Autodesk Inventor part; units mm, degrees
ref_plane "YZ Plane" through (0, 0, 0) normal (1, 0, 0) x (0, 1, 0)
ref_plane "XZ Plane" through (0, 0, 0) normal (0, 1, 0) x (-1, 0, 0)
ref_plane "XY Plane" through (0, 0, 0) normal (0, 0, 1) x (1, 0, 0)
sketch "Boceto1" plane through (0, 0, 0) normal (0, 0, 1) x (1, 0, 0)
  line L0 (-13.5, 62) -> (13.5, 62)
  line L1 (13.5, 62) -> (13.5, 0)
  line L2 (13.5, 0) -> (-13.5, 0)
  line L3 (-13.5, 0) -> (-13.5, 62)
  line L4 (0, 0) -> (0, 62) construction
  line L5 (0, 40.815) -> (8.5, 35.9075)
  line L6 (8.5, 35.9075) -> (8.5, 26.0925)
  line L7 (8.5, 26.0925) -> (0, 21.185)
  line L8 (0, 21.185) -> (-8.5, 26.0925)
  line L9 (-8.5, 26.0925) -> (-8.5, 35.9075)
  line L10 (-8.5, 35.9075) -> (0, 40.815)
  line L11 (-8.5, 35.9075) -> (-13.5, 35.9075) construction
  line L12 (8.5, 35.9075) -> (13.5, 35.9075) construction
  point P0 (0, 31)
  dimension "d20" = 17
  dimension "d21" = 5
  dimension "d22" = 27
  dimension "d23" = 62
extrude "Extrusión1" add sketch "Boceto1" along normal blind 6
sketch "Boceto2" plane through (0, 0, 0) normal (0, 0, -1) x (-1, 0, 0)
  line L0 (-8.5, 26.0925) -> (-8.5, 35.9075)
  line L1 (-8.5, 35.9075) -> (0, 40.815)
  line L2 (0, 40.815) -> (8.5, 35.9075)
  line L3 (8.5, 35.9075) -> (8.5, 26.0925)
  line L4 (8.5, 26.0925) -> (0, 21.185)
  line L5 (0, 21.185) -> (-8.5, 26.0925)
  line L6 (13.5, 62) -> (-13.5, 62)
  line L7 (-13.5, 62) -> (-13.5, 0)
  line L8 (-13.5, 0) -> (13.5, 0)
  line L9 (13.5, 0) -> (13.5, 62)
  point P0 (0, 0)
extrude "Extrusión2" add sketch "Boceto2" along normal blind 6 contours L0 L1 L2 L3 L4 L5 | L9 L8 L7 L6
sketch "Boceto3" plane through (0, 0, -6) normal (0, 0, -1) x (-1, 0, 0)
  line L0 (0, 0) -> (0, 62) construction
  line L1 (-13.5, 62) -> (13.5, 62)
  circle A0 centre (0, 31) radius 5.5
  dimension "d18" = 11
extrude "Extrusión3" cut sketch "Boceto3" against normal up to next
sketch "Boceto5" plane through (0, 0, 6) normal (0, 0, 1) x (1, 0, 0)
  line L0 (-13.5, 0) -> (-13.5, 62)
  line L1 (13.5, 62) -> (13.5, 0)
  line L2 (-13.5, 0) -> (13.5, 0)
  line L3 (13.5, 0) -> (13.5, 12)
  line L4 (13.5, 12) -> (-13.5, 12)
  line L5 (-13.5, 12) -> (-13.5, 0)
  line L6 (13.5, 62) -> (-13.5, 62)
  line L7 (-13.5, 62) -> (13.5, 62)
  line L8 (13.5, 62) -> (13.5, 50)
  line L9 (13.5, 50) -> (-13.5, 50)
  line L10 (-13.5, 50) -> (-13.5, 62)
  line L11 (-17.3027, 31) -> (12.0796, 31) construction
  line L12 (-8.5, 26.0925) -> (-8.5, 35.9075)
  point P0 (0, 0)
  point P1 (-8.5, 31)
  dimension "d24" = 12
extrude "Extrusión4" add sketch "Boceto5" along normal blind 115 contours L0 L4 L1 L2 | L0 L6 L1 L9
sketch "Boceto9" plane through (-13.5, 0, -6) normal (0, -1, 0) x (1, 0, 0)
  circle A0 centre (13.5, 110) radius 5
  line L0 (0, 127) -> (27, 127)
  line L1 (13.5, 110) -> (13.5, 115)
  line L2 (13.5, 115) -> (13.5, 127)
  line L3 (0, 127) -> (27, 127)
  point P0 (13.5, 6)
  dimension "d25" = 10
  dimension "d32" = 12
extrude "Extrusión8" cut sketch "Boceto9" against normal up to surface (12 mm away)
sketch "Boceto10" plane through (0, 0, -6) normal (0, 0, -1) x (-1, 0, 0)
  circle A0 centre (0, 31) radius 11
  circle A1 centre (0, 31) radius 5.5
  point P0 (0, 0)
  dimension "d29" = 22
extrude "Extrusión9" cut sketch "Boceto10" against normal blind 2.5
sketch "Boceto11" plane through (-13.5, 12, 6) normal (0, 1, 0) x (1, 0, 0)
  line L0 (21.5, -106) -> (5.5, -106) construction
  line L1 (5.5, -106) -> (5.5, -90) construction
  line L2 (5.5, -90) -> (21.5, -90) construction
  line L3 (21.5, -90) -> (21.5, -106) construction
  line L4 (5.5, -106) -> (21.5, -90) construction
  circle A0 centre (13.5, -98) radius 8 construction
  circle A1 centre (13.5, -98) radius 11.3137
  line L5 (27, 0) -> (27, -115)
  circle A2 centre (13.5, -98) radius 5
  point P0 (13.5, 6)
  dimension "d45" = 16
extrude "Extrusión10" cut sketch "Boceto11" against normal blind 3 contours A1 | A2
sketch "Boceto12" plane through (-13.5, 0, -6) normal (0, -1, 0) x (1, 0, 0)
  circle A0 centre (13.5, 110) radius 11.3137
  line L0 (0, 127) -> (0, 0)
  point P0 (13.5, 6)
extrude "Extrusión11" cut sketch "Boceto12" against normal blind 3
sketch "Boceto14" plane through (-13.5, 62, -6) normal (0, 1, 0) x (1, 0, 0)
  circle A0 centre (13.5, -110) radius 5
  circle A1 centre (13.5, -110) radius 5
  point P0 (13.5, -6)
  dimension "d38" = 10
extrude "Extrusión12" cut sketch "Boceto14" against normal up to next
sketch "Boceto15" plane through (-13.5, 50, 6) normal (0, -1, 0) x (1, 0, 0)
  circle A0 centre (13.5, 98) radius 5
  circle A1 centre (13.5, 98) radius 12
  point P0 (13.5, -6)
  dimension "d41" = 24
extrude "Extrusión13" cut sketch "Boceto15" against normal blind 8
fillet "Empalme4" radius 12 4 edges at (13.5, 56, 121) (-13.5, 56, 121) (13.5, 6, 121) (-13.5, 6, 121)
fillet "Empalme5" radius 12 2 edges at (0, 0, -6) (0, 62, -6)
fillet "Empalme6" radius 12 2 edges at (0, 12, 6) (0, 50, 6)
CAD build for the part. Positions are in the model's coordinates, mm. A direction names the side the tool comes from. Round coordinates to 2 decimals unless told otherwise and drop trailing zeros. Write each loop counter-clockwise with the first axis right and the second up, starting at its lowest first coordinate (ties: lowest second). Pieces come first, ordered by that corner, then holes. Notation, with made-up numbers: M 31,47 L 57,47 A16 cw 57,74 Z; hole C -1.5,48 d9. An arc over 180 degrees is marked long. Use a Markdown table: item, result. Add a question column.
1. Drill centre lines: probe 1 along Y at (x, z) = (-5.5, 52.5); probe 2 along X at (y, z) = (10.05, 104); probe 3 along Y at (x, z) = (-1.5, 95). Where is each one in solid material? Low to high.
2. Slice it at C-C on z = 47.5. Give the cut face in (x, y).
3. Pull direction X, two halves, no side cores. Call faces 6 (the face through (-12, 31, -6)), 7 (the face through (-0.2, 58, 98.8)), 8 (the face through (-10.08, 56.08, 117.39)): released by +X, released by -X, zero draft, split by the parting line, or undercut.
4. Slice it at B-B on z = 104. Give the cut face in (x, y).
5. Flat gauge pins, fed straight in: P1, Ø7, axis at x = 5.5, z = 98.5, coming from the -Y side; P2, Ø7, axis at x = 11, y = 31, coming from the +Z side; P3, Ø6.5, axis at x = 0, y = 31, coming from the +Z side. Where does each tip first touch, or does it go through?
6. 3-axis set-ups, long thin cutter, end or side, ignore diameter. For faces 1 (the face through (8.5, 31, 3)), 2 (the face through (0, 6, 121)), 3 (the face through (0, 12, 57)), 4 (the face through (-2.453, 1.479, 92.955)), 5 (the face through (0, 0, 63)): which of +Z, -Z, +X, -X, +Y, -Y reach the whole face in a straight line?
7. Slice it at D-D on y = 22.5. Give the cut face in (x, z).
8. Slice it at A-A on y = 31. Give the cut face in (x, z).
Reply:
| question | item | result |
|---|---|---|
| 1 | probe 1 | y = 0 to 12, 50 to 62 |
| 1 | probe 2 | x = -13.5 to -11.31, 11.31 to 13.5 |
| 1 | probe 3 | y = 3 to 9, 58 to 62 |
| 2 | outline | M -13.5,0 L 13.5,0 L 13.5,12 L -13.5,12 Z; M -13.5,50 L 13.5,50 L 13.5,62 L -13.5,62 Z |
| 3 | face 6 | zero draft |
| 3 | face 7 | undercut |
| 3 | face 8 | released by -X |
| 4 | outline | M -13.5,0 L -11.31,0 L -11.31,3 L -5,3 L -5,9 L -11.31,9 L -11.31,12 L -13.5,12 Z; M -13.5,50 L -12,50 L -12,58 L -5,58 L -5,62 L -13.5,62 Z; M 5,3 L 11.31,3 L 11.31,0 L 13.5,0 L 13.5,12 L 11.31,12 L 11.31,9 L 5,9 Z; M 5,58 L 12,58 L 12,50 L 13.5,50 L 13.5,62 L 5,62 Z |
| 5 | P1 | stops at y = 3 |
| 5 | P2 | stops at z = 6 |
| 5 | P3 | passes through |
| 6 | face 1 | +Z |
| 6 | face 2 | +Z, +X, -X, +Y, -Y |
| 6 | face 3 | +Z, +X, -X |
| 6 | face 4 | -Y |
| 6 | face 5 | +Z, -Z, +X, -X, -Y |
| 7 | outline | M -13.5,-6 L -6.98,-6 L -6.98,-3.5 L 6.98,-3.5 L 6.98,-6 L 13.5,-6 L 13.5,6.09 L 2.28,6.09 L 2.28,0 L -2.28,0 L -2.28,6.09 L -13.5,6.09 Z |
| 8 | outline | M -13.5,-6 L -11,-6 L -11,-3.5 L -5.5,-3.5 L -5.5,0 L -8.5,0 L -8.5,6 L -13.5,6 Z; M 5.5,-3.5 L 11,-3.5 L 11,-6 L 13.5,-6 L 13.5,6 L 8.5,6 L 8.5,0 L 5.5,0 Z |
